Geometry: final body of the model. Coordinates: model frame, mm. Face numbers are marked on the shaded views. A direction names the side the tool comes from. Round coordinates to 2 decimals unless told otherwise and drop trailing zeros. Loops run counter-clockwise (first coordinate to the right, second up) from the corner with the lowest first, then second, coordinate; pieces in that order, holes last. Notation, with made-up numbers: M -19.75,37 L 22.25,37 A20 cw 22.25,52 Z; hole C 59,-39.75 d9. An arc over 180 degrees is marked long. Write each question's results on one line, items separated by ' | '.
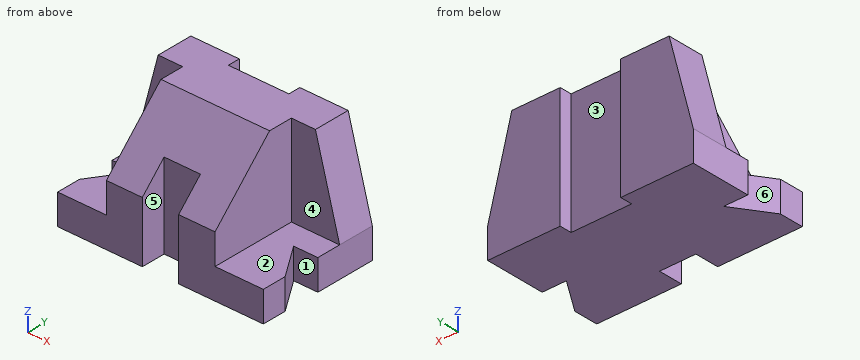
```python
from build123d import *

# Parameters (mm, degrees)
PAD_DEPTH       = 100
SKETCH002_W     = 61.512183
SKETCH002_H     = 94.726295
SKETCH002_W_2   = 51.517512
SKETCH002_H_2   = 91.373596
POCKET_DEPTH    = 75
POCKET001_DEPTH = 129.705213
POCKET002_DEPTH = 30.001


with BuildPart() as part:
    # Sketch → Pad (new body)
    with BuildSketch(Plane.XY):
        Polygon((-85, 0), (-25, 0), (-25, -10), (25, -10), (25, 0), (85, 0), (85, -50), (65, -50), (85, -80), (85, -100), (15, -100), (15, -80), (-15, -80), (-15, -100), (-85, -100), (-85, -80), (-65, -50), (-85, -50), align=None)
    extrude(amount=PAD_DEPTH)

    # Sketch002 → Pocket (cut)
    with BuildSketch(Plane.XY.offset(100)):
        with Locations((75.860517, -77.363147)):
            Rectangle(SKETCH002_W, SKETCH002_H)
        with Locations((-70.462969, -75.686798)):
            Rectangle(SKETCH002_W_2, SKETCH002_H_2)
    extrude(amount=-POCKET_DEPTH, mode=Mode.SUBTRACT)

    # Sketch003 → Pocket001 (cut, through all)
    with BuildSketch(Plane(origin=(-44.704213, 0, 0), x_dir=(0, -1, 0), z_dir=(-1, 0, 0))):
        Polygon((100, 100), (100, 50), (50, 100), align=None)
    extrude(amount=-POCKET001_DEPTH, mode=Mode.SUBTRACT)

    # Sketch004 → Pocket002 (cut, through all)
    with BuildSketch(Plane.XZ.offset(30)):
        Polygon((-85, 100), (-65, 100), (-85, 25), align=None)
        Polygon((85, 100), (65, 100), (85, 25), align=None)
    extrude(amount=-POCKET002_DEPTH, mode=Mode.SUBTRACT)


solid = part.part
```
1. Draft query along Y for the marked faces 1, 2 and 3. Return one class per face: pulls with the +Y half, pulls with the -Y half, needs draft (parallel to the pull), parting line crosses it, or undercut.
Answer key:
face 1: undercut | face 2: needs draft | face 3: pulls with the +Y half
2. Section C-C (z = 16.5). Output: boundary loops of the cut face in (x, y).
Answer key:
outline: M -85,-100 L -15,-100 L -15,-80 L 15,-80 L 15,-100 L 85,-100 L 85,-80 L 65,-50 L 85,-50 L 85,0 L 25,0 L 25,-10 L -25,-10 L -25,0 L -85,0 L -85,-50 L -65,-50 L -85,-80 Z
3. Ray query, probe 1 along X at (y, z) = (-85, 41); probe 2 along X at (y, z) = (-6, 4); probe 3 along Z at (x, y) = (-59, -75). Return the intervals inside material, ascending.
Answer key:
probe 1: x = -44.7 to -15, 15 to 45.1 | probe 2: x = -85 to -25, 25 to 85 | probe 3: z = 0 to 25
4. Section B-B (y = -42). Output: boundary loops of the cut face in (x, z).
Answer key:
outline: M -85,0 L 85,0 L 85,25 L 45.1,25 L 45.1,100 L -44.7,100 L -44.7,25 L -85,25 Z
5. Section A-A (y = -91.5). Output: boundary loops of the cut face in (x, z).
Answer key:
outline: M -85,0 L -15,0 L -15,58.5 L -44.7,58.5 L -44.7,25 L -85,25 Z; M 15,0 L 85,0 L 85,25 L 45.1,25 L 45.1,58.5 L 15,58.5 Z
6. Section D-D (x = 70.5). Output: boundary loops of the cut face in (y, z) (3 decimals).
Answer key:
outline: M -100,0 L -58.25,0 L -58.25,25 L -100,25 Z; M -50,0 L 0,0 L 0,79.375 L -30,79.375 L -30,25 L -50,25 Z
7. Pin query (flat end, axial travel): P1, Ø3, axis at y = -6, z = 35, coming from the -X side; P2, Ø15, axis at x = 5.5, z = 64, coming from the +Y side; P3, Ø5, axis at x = 66, y = -71.5, coming from the -Z side; P4, Ø3, axis at y = -6, z = 63.5, coming from the +X side. Return the tip coordinate at first contact, or that it passes through.
Answer key:
P1: stops at x = -82.73 | P2: stops at y = -10 | P3: stops at z = 0 | P4: stops at x = 75.13
8. Access query for the marked faces 4, 5 and 6. Directions: +Z, -Z, +X, -X, +Y, -Y. A direction counts if a zero-diameter tool reaches every point of the face in a straight line with its end or side. Return the directions, or none.
Answer key:
face 4: +Z, +X, -Y | face 5: +Z, -Z, -Y | face 6: +Z, -Z, -X
